The listing builds one solid part. Answer for the finished solid, in the listing's coordinates (mm). A direction names the side the tool comes from. Coordinates: 2 decimals unless noted, no trailing zeros. Order: outer loops, then holes, each group sorted by start corner. A loop starts at its lowest first (then second) coordinate and runs counter-clockwise, first axis right, second up. Notation, with made-up numbers: (78, -24) - (109, -24) arc R27 cw to (109, 6) - close; hole circle Ø11 at (0.25, 32.5). An arc over 180 degrees is marked (long way). One line per item, written item: value. Start each with the question number.
```python
from build123d import *

# Parameters (mm, degrees)
SKETCH1_W               = 76.2
SKETCH1_H               = 17.526
BOSS_EXTRUDE1_DEPTH     = 3.175
SKETCH2_W               = 17.78
SKETCH2_H               = 3.175
CUT_EXTRUDE1_DEPTH      = 79.2539539
MIRROR2_COPY_1_SKETCH_W = 17.78
MIRROR2_COPY_1_SKETCH_H = 3.175
MIRROR2_COPY_1_DEPTH    = 79.2539539
HOLE1_D                 = 5.08
SKETCH5_W               = 3.175
SKETCH5_H               = 17.526
CUT_EXTRUDE2_DEPTH      = 3.81
SKETCH6_W               = 3.175
SKETCH6_H               = 17.526
CUT_EXTRUDE3_DEPTH      = 3.81


with BuildPart() as part:
    # Sketch1 → Boss-Extrude1 (new body)
    with BuildSketch(Plane.XY):
        with Locations((38.1, -8.763)):
            Rectangle(SKETCH1_W, SKETCH1_H)
    extrude(amount=BOSS_EXTRUDE1_DEPTH)

    # Sketch2 → Cut-Extrude1 (cut, through all)
    with BuildSketch(Plane.XY.offset(3.175)):
        with Locations((20.32, -1.5875)):
            Rectangle(SKETCH2_W, SKETCH2_H)
    cut_extrude1 = extrude(amount=-CUT_EXTRUDE1_DEPTH, mode=Mode.SUBTRACT)

    # Mirror1: Cut-Extrude1 across plane
    add(cut_extrude1.mirror(Plane.ZX.offset(-8.763)), mode=Mode.SUBTRACT)

    # Mirror2: Cut-Extrude1 across plane
    add(cut_extrude1.mirror(Plane(origin=(38.1, 0, 0), x_dir=(0, 0, 1), z_dir=(1, 0, 0))), mode=Mode.SUBTRACT)

    # Mirror2 copy 1 sketch → Mirror2 copy 1 (cut, through all)
    with BuildSketch(Plane(origin=(76.2, -17.526, 3.175), x_dir=(-1, 0, 0), z_dir=(0, 0, 1))):
        with Locations((20.32, -1.5875)):
            Rectangle(MIRROR2_COPY_1_SKETCH_W, MIRROR2_COPY_1_SKETCH_H)
    extrude(amount=-MIRROR2_COPY_1_DEPTH, mode=Mode.SUBTRACT)

    # Hole1 (through all)
    with Locations(Plane.XY.offset(3.175)):
        with Locations((15.24, -8.763), (38.1, -8.763), (26.67, -8.763), (49.53, -8.763), (60.96, -8.763)):
            Hole(HOLE1_D / 2)

    # Sketch5 → Cut-Extrude2 (cut)
    with BuildSketch(Plane.ZY):
        with Locations((1.5875, -8.763)):
            Rectangle(SKETCH5_W, SKETCH5_H)
    extrude(amount=-CUT_EXTRUDE2_DEPTH, mode=Mode.SUBTRACT)

    # Sketch6 → Cut-Extrude3 (cut)
    with BuildSketch(Plane(origin=(76.2, 0, 0), x_dir=(0, 0, -1), z_dir=(1, 0, 0))):
        with Locations((-1.5875, -8.763)):
            Rectangle(SKETCH6_W, SKETCH6_H)
    extrude(amount=-CUT_EXTRUDE3_DEPTH, mode=Mode.SUBTRACT)


solid = part.part
```
(1) For faces 4 (the face through (20, -3.175, 2)), 5 (the face through (38, -17.526, 2)), 6 (the face through (46.99, -16, 2)), determine the directions among +Z, -Z, +X, -X, +Y, -Y from which every point of the face is accessible in a straight line to the end or side of a thin tool.
(2) For a pull along Y with two mould halves and no side action, classify faces 1 (the face through (29.208, -8.651, 1.565)), 2 (the face through (29.21, -16, 2)), 3 (the face through (8, -17.526, 2)) as pulls with the +Y half, pulls with the -Y half, needs draft (parallel to the pull), parting line crosses it, or undercut.
(3) The part is cut by section A-A on x = 38.1. Determine the outline of the cut face in (y, z) (3 decimals), plus the area to 3 significant figures.
(4) The part is cut by section D-D on z = 2.3. Determine the outline of the cut face in (x, y) (3 decimals).
(5) The part is cut by section B-B on y = -7.75. Determine the outline of the cut face in (x, z) (3 decimals), plus the area to 3 significant figures.
(6) Consider probe 1 along X at (y, z) = (-15.5, 1.9); probe 2 along Y at (x, z) = (15.24, 0.8) (3 decimals); probe 3 along X at (y, z) = (-7, 3). Determine where each line is inside the solid, lowest interval first.
(7) The part is cut by section C-C on x = 15.24. Determine the outline of the cut face in (y, z) (3 decimals), plus the area to 3 significant figures.
Completed:
1. face 4: +Z, -Z, +Y
1. face 5: +Z, -Z, +X, -X, -Y
1. face 6: +Z, -Z, -Y
2. face 1: undercut
2. face 2: needs draft
2. face 3: pulls with the -Y half
3. outline: (-17.526, 0) - (-11.303, 0) - (-11.303, 3.175) - (-17.526, 3.175) - close; (-6.223, 0) - (0, 0) - (0, 3.175) - (-6.223, 3.175) - close
3. area: 39.5 mm2
4. outline: (3.81, -17.526) - (11.43, -17.526) - (11.43, -14.351) - (29.21, -14.351) - (29.21, -17.526) - (46.99, -17.526) - (46.99, -14.351) - (64.77, -14.351) - (64.77, -17.526) - (72.39, -17.526) - (72.39, 0) - (64.77, 0) - (64.77, -3.175) - (46.99, -3.175) - (46.99, 0) - (29.21, 0) - (29.21, -3.175) - (11.43, -3.175) - (11.43, 0) - (3.81, 0) - close; hole circle Ø5.08 at (15.24, -8.763); hole circle Ø5.08 at (26.67, -8.763); hole circle Ø5.08 at (38.1, -8.763); hole circle Ø5.08 at (49.53, -8.763); hole circle Ø5.08 at (60.96, -8.763)
5. outline: (3.81, 0) - (12.911, 0) - (12.911, 3.175) - (3.81, 3.175) - close; (17.569, 0) - (24.341, 0) - (24.341, 3.175) - (17.569, 3.175) - close; (28.999, 0) - (35.771, 0) - (35.771, 3.175) - (28.999, 3.175) - close; (40.429, 0) - (47.201, 0) - (47.201, 3.175) - (40.429, 3.175) - close; (51.859, 0) - (58.631, 0) - (58.631, 3.175) - (51.859, 3.175) - close; (63.289, 0) - (72.39, 0) - (72.39, 3.175) - (63.289, 3.175) - close
5. area: 144 mm2
6. probe 1: x = 3.81 to 11.43, 29.21 to 46.99, 64.77 to 72.39
6. probe 2: y = -14.351 to -11.303, -6.223 to -3.175
6. probe 3: x = 3.81 to 13.41, 17.07 to 24.84, 28.5 to 36.27, 39.93 to 47.7, 51.36 to 59.13, 62.79 to 72.39
7. outline: (-14.351, 0) - (-11.303, 0) - (-11.303, 3.175) - (-14.351, 3.175) - close; (-6.223, 0) - (-3.175, 0) - (-3.175, 3.175) - (-6.223, 3.175) - close
7. area: 19.4 mm2
